Read the model definition and answer for the solid it produces. Units are mm, in the model's axes. A direction names the side the tool comes from. Coordinates: 2 decimals unless noted, no trailing zeros. Loops run counter-clockwise (first coordinate to the right, second up) from the corner with the lowest first, then second, coordinate; pieces in that order, holes last. Notation, with made-up numbers: M 47,-7.75 L 86,-7.75 A15 cw 86,16.25 Z; hole C 1.5,7 d6. An arc over 180 degrees is marked long. One line per item, written item: value. Start each with the question number.
1. The part is cut by section C-C (z = 29). Write down the section's boundary in (x, y).
2. The part is cut by section A-A (x = 52.5). Write down the section's boundary in (y, z), then the cut area to 3 significant figures.
3. For faces 1 (the face through (45.4, -2.5, 23.6)), 2 (the face through (15.7, -12, 42.3)), determine the directions among +Z, -Z, +X, -X, +Y, -Y from which every point of the face is accessible in a straight line to the end or side of a thin tool.
4. The part is cut by section D-D (x = 29). Write down the section's boundary in (y, z).
5. The part is cut by section B-B (y = -4). Write down the section's boundary in (x, z).
6. Consider probe 1 along Z at (x, y) = (52.5, -6.5); probe 2 along X at (y, z) = (-2.5, 5); probe 3 along Z at (x, y) = (4, -9). Determine where each line is inside the solid, lowest interval first.
```python
from build123d import *

# Parameters (mm, degrees)
F0_W     = 58
F0_H     = 58
F0_R     = 17
F1_DEPTH = 12
F2_R     = 18.5
F2_R_2   = 17
F3_DEPTH = 9.5
F5_D     = 6.8


with BuildPart() as f1:
    # F0 (on Front) → F1 (new body)
    with BuildSketch(Plane.XZ):
        with Locations((29, 29)):
            Rectangle(F0_W, F0_H)
        with Locations((29, 29)):
            Circle(F0_R, mode=Mode.SUBTRACT)
    extrude(amount=F1_DEPTH)

    # F2 (on face) → F3 (cut)
    with BuildSketch(Plane.XZ.offset(12)):
        with Locations((29, 29)):
            Circle(F2_R)
        with Locations((29, 29)):
            Circle(F2_R_2, mode=Mode.SUBTRACT)
    extrude(amount=-F3_DEPTH, mode=Mode.SUBTRACT)

    # F5 (through all)
    with Locations(Plane.XZ.offset(12)):
        with Locations((5.5, 52.5), (52.5, 52.5), (52.5, 5.5), (5.5, 5.5)):
            Hole(F5_D / 2)


solid = f1.part
```
Answer block:
1. outline: M 0,-12 L 10.5,-12 L 10.5,-2.5 L 12,-2.5 L 12,0 L 0,0 Z; M 46,-2.5 L 47.5,-2.5 L 47.5,-12 L 58,-12 L 58,0 L 46,0 Z
2. outline: M -12,0 L 0,0 L 0,2.1 L -12,2.1 Z; M -12,8.9 L 0,8.9 L 0,49.1 L -12,49.1 Z; M -12,55.9 L 0,55.9 L 0,58 L -12,58 Z
2. area: 533 mm2
3. face 1: -Y
3. face 2: +Z, -Z, +X, -X, -Y
4. outline: M -12,0 L 0,0 L 0,12 L -2.5,12 L -2.5,10.5 L -12,10.5 Z; M -12,47.5 L -2.5,47.5 L -2.5,46 L 0,46 L 0,58 L -12,58 Z
5. outline: M 0,0 L 58,0 L 58,58 L 0,58 Z; hole C 5.5,5.5 d6.8; hole C 5.5,52.5 d6.8; hole C 29,29 d37; hole C 52.5,5.5 d6.8; hole C 52.5,52.5 d6.8
6. probe 1: z = 0 to 2.1, 8.9 to 49.1, 55.9 to 58
6. probe 2: x = 0 to 2.14, 8.86 to 49.14, 55.86 to 58
6. probe 3: z = 0 to 2.45, 8.55 to 49.45, 55.55 to 58
